Verification items for the finished model (mm, model axes). A direction names the side the tool comes from. Coordinates: 2 decimals unless noted, no trailing zeros. Write each loop counter-clockwise with the first axis right and the second up, starting at its lowest first coordinate (ties: lowest second). Pieces come first, ordered by that corner, then holes. Notation, with made-up numbers: M 37,25.25 L 46,25.25 A17 cw 46,34.25 Z; hole C 28.5,-21.5 d3. An arc over 180 degrees is marked long. Answer in a Markdown table with one row per item.
from build123d import *

# Parameters (mm, degrees)
SKETCH1_W                      = 100
SKETCH1_H                      = 100
BASE_FLANGE1_DEPTH             = 7
EDGE_FLANGE1_STRIP_W           = 29.4732
EDGE_FLANGE1_STRIP_H           = 7
EDGE_FLANGE1_STRIP_CUT_DEPTH   = 100
EDGE_FLANGE1_STRIP_2_W         = 29.4732
EDGE_FLANGE1_STRIP_2_H         = 7
EDGE_FLANGE1_STRIP_CUT_2_DEPTH = 100
EDGE_FLANGE1_DEPTH             = 100
EDGE_FLANGE1_BEND_DEPTH        = 100
SHEET_START                    = -3.5
SHEET_METAL_GUSSET13_DEPTH     = 7
SHEET_START_2                  = -10.5
SHEET_METAL_GUSSET13_2_DEPTH   = 21
SHEET_METAL_GUSSET13_3_DEPTH   = 7
SHEET_START_3                  = 3.5
SHEET_METAL_GUSSET13_4_DEPTH   = 7
SHEET_METAL_GUSSET14_DEPTH     = 7
SHEET_METAL_GUSSET14_2_DEPTH   = 21
SHEET_METAL_GUSSET14_3_DEPTH   = 7
SHEET_METAL_GUSSET14_4_DEPTH   = 7
EDGE_FLANGE3_STRIP_W           = 29.4732
EDGE_FLANGE3_STRIP_H           = 7
EDGE_FLANGE3_STRIP_CUT_DEPTH   = 100
EDGE_FLANGE3_DEPTH             = 100
F_16_0MM_DOWEL_HOLE1_D         = 16


# Read off the part's stored shape, not the designer's step: Sheet Metal Gusset13, Sheet Metal Gusset14
# Sheet-metal steps are written as plain solids
with BuildPart() as part:
    # Sketch1 → Base-Flange1 (new body)
    with BuildSketch(Plane(origin=(0, 0, 0), x_dir=(1, 0, 0), z_dir=(0, 1, 0))):
        Rectangle(SKETCH1_W, SKETCH1_H)
    extrude(amount=-BASE_FLANGE1_DEPTH)

    # Edge-Flange1 strip (across the edge) → Edge-Flange1 strip cut (cut)
    with BuildSketch(Plane(origin=(-50, 0, -50), x_dir=(1, 0, 0), z_dir=(0, 0, 1))):
        with Locations((-7, -3.5)):
            Rectangle(EDGE_FLANGE1_STRIP_W, EDGE_FLANGE1_STRIP_H)
    extrude(amount=EDGE_FLANGE1_STRIP_CUT_DEPTH, mode=Mode.SUBTRACT)

    # Edge-Flange1 strip 2 (across the edge) → Edge-Flange1 strip cut 2 (cut)
    with BuildSketch(Plane(origin=(50, 0, 50), x_dir=(-1, 0, 0), z_dir=(0, 0, -1))):
        with Locations((-7, -3.5)):
            Rectangle(EDGE_FLANGE1_STRIP_2_W, EDGE_FLANGE1_STRIP_2_H)
    extrude(amount=EDGE_FLANGE1_STRIP_CUT_2_DEPTH, mode=Mode.SUBTRACT)

    # Edge-Flange1 section (across the edge) → Edge-Flange1 (add)
    with BuildSketch(Plane(origin=(-50, 0, -50), x_dir=(1, 0, 0), z_dir=(0, 0, 1))):
        with BuildLine():
            Line((0, 0.7366), (0, 43))
            Line((0, 43), (7, 43))
            Line((7, 43), (7, 0.7366))
            ThreePointArc((7, 0.7366), (7.215745145, 0.215745145), (7.7366, 0))
            Line((7.7366, 0), (7.7366, -7))
            ThreePointArc((7.7366, -7), (2.265997677, -4.734002323), (0, 0.7366))
        make_face()
    extrude(amount=EDGE_FLANGE1_DEPTH)

    # Edge-Flange1 section 2 (across the edge) → Edge-Flange1 bend (add)
    with BuildSketch(Plane(origin=(50, 0, 50), x_dir=(-1, 0, 0), z_dir=(0, 0, -1))):
        with BuildLine():
            Line((0, 0.7366), (0, 43))
            Line((0, 43), (7, 43))
            Line((7, 43), (7, 0.7366))
            ThreePointArc((7, 0.7366), (7.215745145, 0.215745145), (7.7366, 0))
            Line((7.7366, 0), (7.7366, -7))
            ThreePointArc((7.7366, -7), (2.265997677, -4.734002323), (0, 0.7366))
        make_face()
    extrude(amount=EDGE_FLANGE1_BEND_DEPTH)

    # Sheet Metal Gusset13 outline → Sheet Metal Gusset13 (cut)
    with BuildSketch(Plane.XY.offset(SHEET_START)):
        with BuildLine():
            Line((42.2634, 0), (38.325869023, 0))
            Line((38.325869023, 0), (31.325869023, -7))
            Line((31.325869023, -7), (42.2634, -7))
            ThreePointArc((42.2634, -7), (47.734002323, -4.734002323), (50, 0.7366))
            Line((50, 0.7366), (50, 11.674130977))
            Line((50, 11.674130977), (43, 4.674130977))
            Line((43, 4.674130977), (43, 0.7366))
            ThreePointArc((43, 0.7366), (42.784254855, 0.215745145), (42.2634, 0))
        make_face()
    extrude(amount=SHEET_METAL_GUSSET13_DEPTH, mode=Mode.SUBTRACT)

    # Sheet Metal Gusset13 2 outline → Sheet Metal Gusset13 2 (add)
    with BuildSketch(Plane.XY.offset(SHEET_START_2)):
        Polygon((43, 14.573625914), (28.426374086, 0), (38.325869023, 0), (43, 4.674130977), align=None)
    extrude(amount=SHEET_METAL_GUSSET13_2_DEPTH)

    # Sheet Metal Gusset13 3 outline → Sheet Metal Gusset13 3 (add)
    with BuildSketch(Plane.XY.offset(SHEET_START_2)):
        with BuildLine():
            Line((43, 4.674130977), (38.325869023, 0))
            Line((38.325869023, 0), (42.2634, 0))
            ThreePointArc((42.2634, 0), (42.784254855, 0.215745145), (43, 0.7366))
            Line((43, 0.7366), (43, 4.674130977))
        make_face()
    extrude(amount=SHEET_METAL_GUSSET13_3_DEPTH)

    # Sheet Metal Gusset13 4 outline → Sheet Metal Gusset13 4 (add)
    with BuildSketch(Plane.XY.offset(SHEET_START_3)):
        with BuildLine():
            Line((43, 4.674130977), (38.325869023, 0))
            Line((38.325869023, 0), (42.2634, 0))
            ThreePointArc((42.2634, 0), (42.784254855, 0.215745145), (43, 0.7366))
            Line((43, 0.7366), (43, 4.674130977))
        make_face()
    extrude(amount=SHEET_METAL_GUSSET13_4_DEPTH)

    # Sheet Metal Gusset14 outline → Sheet Metal Gusset14 (cut)
    with BuildSketch(Plane.XY.offset(SHEET_START)):
        with BuildLine():
            Line((-43, 0.7366), (-43, 4.674130977))
            Line((-43, 4.674130977), (-50, 11.674130977))
            Line((-50, 11.674130977), (-50, 0.7366))
            ThreePointArc((-50, 0.7366), (-47.734002323, -4.734002323), (-42.2634, -7))
            Line((-42.2634, -7), (-31.325869023, -7))
            Line((-31.325869023, -7), (-38.325869023, 0))
            Line((-38.325869023, 0), (-42.2634, 0))
            ThreePointArc((-42.2634, 0), (-42.784254855, 0.215745145), (-43, 0.7366))
        make_face()
    extrude(amount=SHEET_METAL_GUSSET14_DEPTH, mode=Mode.SUBTRACT)

    # Sheet Metal Gusset14 2 outline → Sheet Metal Gusset14 2 (add)
    with BuildSketch(Plane.XY.offset(SHEET_START_2)):
        Polygon((-28.426374086, 0), (-43, 14.573625914), (-43, 4.674130977), (-38.325869023, 0), align=None)
    extrude(amount=SHEET_METAL_GUSSET14_2_DEPTH)

    # Sheet Metal Gusset14 3 outline → Sheet Metal Gusset14 3 (add)
    with BuildSketch(Plane.XY.offset(SHEET_START_2)):
        with BuildLine():
            Line((-38.325869023, 0), (-43, 4.674130977))
            Line((-43, 4.674130977), (-43, 0.7366))
            ThreePointArc((-43, 0.7366), (-42.784254855, 0.215745145), (-42.2634, 0))
            Line((-42.2634, 0), (-38.325869023, 0))
        make_face()
    extrude(amount=SHEET_METAL_GUSSET14_3_DEPTH)

    # Sheet Metal Gusset14 4 outline → Sheet Metal Gusset14 4 (add)
    with BuildSketch(Plane.XY.offset(SHEET_START_3)):
        with BuildLine():
            Line((-38.325869023, 0), (-43, 4.674130977))
            Line((-43, 4.674130977), (-43, 0.7366))
            ThreePointArc((-43, 0.7366), (-42.784254855, 0.215745145), (-42.2634, 0))
            Line((-42.2634, 0), (-38.325869023, 0))
        make_face()
    extrude(amount=SHEET_METAL_GUSSET14_4_DEPTH)

    # Edge-Flange3 strip (across the edge) → Edge-Flange3 strip cut (cut)
    with BuildSketch(Plane(origin=(-50, 43, 50), x_dir=(0, -1, 0), z_dir=(0, 0, -1))):
        with Locations((-7, -3.5)):
            Rectangle(EDGE_FLANGE3_STRIP_W, EDGE_FLANGE3_STRIP_H)
    extrude(amount=EDGE_FLANGE3_STRIP_CUT_DEPTH, mode=Mode.SUBTRACT)

    # Edge-Flange3 section (across the edge) → Edge-Flange3 (add)
    with BuildSketch(Plane(origin=(-50, 43, 50), x_dir=(0, -1, 0), z_dir=(0, 0, -1))):
        with BuildLine():
            Line((0, 0.7366), (0, 58))
            Line((0, 58), (7, 58))
            Line((7, 58), (7, 0.7366))
            ThreePointArc((7, 0.7366), (7.215745145, 0.215745145), (7.7366, 0))
            Line((7.7366, 0), (7.7366, -7))
            ThreePointArc((7.7366, -7), (2.265997677, -4.734002323), (0, 0.7366))
        make_face()
    extrude(amount=EDGE_FLANGE3_DEPTH)

    # Ø16.0mm Dowel Hole1 (through all)
    with Locations(Plane(origin=(0, 36, 0), x_dir=(-1, 0, 0), z_dir=(0, -1, 0))):
        with Locations((79.3683, -25), (79.3683, 25)):
            Hole(F_16_0MM_DOWEL_HOLE1_D / 2)


solid = part.part
1) Tool access check on faces 5 (the face through (-43, 18, -1)), 6 (the face through (39, 4, -10.5)), 7 (the face through (-35.611, 7.185, -0.147)), 8 (the face through (-43, 0, -3.5)), 9 (the face through (40.532, 2.206, -0.049)). Record the directions out of +Z, -Z, +X, -X, +Y, -Y that give a thin tool (end or side, any length) a straight path to the whole face; none if there is none.
Response values:
| item | result |
|---|---|
| face 5 | +Y |
| face 6 | -Z, +Y |
| face 7 | +Z, -Z, +Y |
| face 8 | -X, -Y |
| face 9 | +X, -Y |
2) Depth check by flat-ended pin: pin 1 (4.5 mm diameter, centred on x = -38.5, y = 6.5, fed in from +Z); pin 2 (15 mm diameter, centred on x = -41.5, y = 5.5, fed in from +Z); pin 3 (4 mm diameter, centred on y = 25, z = 21, fed in from -X); pin 4 (16 mm diameter, centred on x = 34.5, y = 8.5, fed in from -Z). Enter the tip coordinate at first touch or a pass-through.
Response values:
| item | result |
|---|---|
| pin 1 | stops at z = 10.5 |
| pin 2 | stops at z = 50 |
| pin 3 | stops at x = -50 |
| pin 4 | stops at z = -10.5 |
3) Sectioned sample at A-A (z = -25). Record the cut outline in (x, y).
Response values:
| item | result |
|---|---|
| outline | M -108,36 L -87.37,36 L -87.37,43 L -108,43 Z; M -71.37,36 L -50.74,36 A0.74 cw -50,35.26 L -50,0.74 A7.74 ccw -42.26,-7 L 42.26,-7 A7.74 ccw 50,0.74 L 50,43 L 43,43 L 43,0.74 A0.74 cw 42.26,0 L -42.26,0 A0.74 cw -43,0.74 L -43,35.26 A7.74 ccw -50.74,43 L -71.37,43 Z |
4) Sectioned sample at C-C (z = -36). Record the cut outline in (x, y).
Response values:
| item | result |
|---|---|
| outline | M -108,36 L -50.74,36 A0.74 cw -50,35.26 L -50,0.74 A7.74 ccw -42.26,-7 L 42.26,-7 A7.74 ccw 50,0.74 L 50,43 L 43,43 L 43,0.74 A0.74 cw 42.26,0 L -42.26,0 A0.74 cw -43,0.74 L -43,35.26 A7.74 ccw -50.74,43 L -108,43 Z |
5) Sectioned sample at D-D (x = 17). Record the cut outline in (y, z), then the cut area to 3 significant figures.
Response values:
| item | result |
|---|---|
| outline | M -7,-50 L 0,-50 L 0,50 L -7,50 Z |
| area | 700 mm² |
6) Sectioned sample at B-B (y = 40). Record the cut outline in (x, z).
Response values:
| item | result |
|---|---|
| outline | M -108,-50 L -44.62,-50 L -44.62,50 L -108,50 Z; M 43,-50 L 50,-50 L 50,50 L 43,50 Z; hole C -79.37,-25 d16; hole C -79.37,25 d16 |
7) Thickness scan on L1, parallel to X at y = 15, z = 2; L2, parallel to Y at x = -6.5, z = -9; L3, parallel to Y at x = -73.5, z = -6.5. Record the ranges inside material, lowest first. Write a range as [from, to].
Response values:
| item | result |
|---|---|
| L1 | x = [-50, -43], [43, 50] |
| L2 | y = [-7, 0] |
| L3 | y = [36, 43] |
8) Release check for a two-part mould opening along Z. For faces 1 (the face through (-1, -7, -1)), 2 (the face through (-87.36, 39.55, 24.65)), 3 (the face through (-39, 4, 10.5)), 4 (the face through (-40.794, 2.468, -0.049)) record: +Z half, -Z half, draft (parallel to the pull), parting line (faces both ways), or undercut.
Response values:
| item | result |
|---|---|
| face 1 | draft |
| face 2 | undercut |
| face 3 | +Z half |
| face 4 | undercut |
